```python
from build123d import *

# Parameters (mm, degrees)
SKETCH_1_W      = 14.7
SKETCH_1_H      = 5.8
EXTRUDE_1_DEPTH = 6


with BuildPart() as part:
    # Эскиз1 → Бобышка-Вытянуть1 (new body)
    with BuildSketch(Plane.XY):
        Polygon((-327.15, -30.4), (327.15, -30.4), (327.15, -17.066666667), (330.45862, -17.066666667), (330.45862, -6.666666667), (327.15, -6.666666667), (327.15, 6.666666667), (330.45862, 6.666666667), (330.45862, 17.066666667), (327.15, 17.066666667), (327.15, 30.4), (-327.15, 30.4), (-330.45862, 30.4), (-330.45862, 16.533333333), (-327.15, 16.533333333), (-327.15, 6.933333333), (-330.45862, 6.933333333), (-330.45862, -6.933333333), (-327.15, -6.933333333), (-327.15, -16.533333333), (-330.45862, -16.533333333), (-330.45862, -30.4), align=None)
        with Locations((-252.05, -2.5)):
            Rectangle(SKETCH_1_W, SKETCH_1_H, mode=Mode.SUBTRACT)
        with Locations((-302.46, -2.5)):
            Rectangle(SKETCH_1_W, SKETCH_1_H, mode=Mode.SUBTRACT)
        with Locations((-201.64, -2.5)):
            Rectangle(SKETCH_1_W, SKETCH_1_H, mode=Mode.SUBTRACT)
        with Locations((-151.23, -2.5)):
            Rectangle(SKETCH_1_W, SKETCH_1_H, mode=Mode.SUBTRACT)
        with Locations((-100.82, -2.5)):
            Rectangle(SKETCH_1_W, SKETCH_1_H, mode=Mode.SUBTRACT)
        with Locations((-50.41, -2.5)):
            Rectangle(SKETCH_1_W, SKETCH_1_H, mode=Mode.SUBTRACT)
        with Locations((0, -2.5)):
            Rectangle(SKETCH_1_W, SKETCH_1_H, mode=Mode.SUBTRACT)
        with Locations((50.41, -2.5)):
            Rectangle(SKETCH_1_W, SKETCH_1_H, mode=Mode.SUBTRACT)
        with Locations((100.82, -2.5)):
            Rectangle(SKETCH_1_W, SKETCH_1_H, mode=Mode.SUBTRACT)
        with Locations((151.23, -2.5)):
            Rectangle(SKETCH_1_W, SKETCH_1_H, mode=Mode.SUBTRACT)
        with Locations((201.64, -2.5)):
            Rectangle(SKETCH_1_W, SKETCH_1_H, mode=Mode.SUBTRACT)
        with Locations((252.05, -2.5)):
            Rectangle(SKETCH_1_W, SKETCH_1_H, mode=Mode.SUBTRACT)
        with Locations((302.46, -2.5)):
            Rectangle(SKETCH_1_W, SKETCH_1_H, mode=Mode.SUBTRACT)
    extrude(amount=EXTRUDE_1_DEPTH)


solid = part.part
```
Part model, mm, in its own coordinate system. Round coordinates to 2 decimals unless told otherwise and drop trailing zeros. One line per question, with ' | ' between items.
(1) Probe line 1 along Y through (x, z) = (-152, 3.4); line 2 along X through (y, z) = (-14, 4); line 3 along X through (y, z) = (-22, 4.55). List the from-to ranges inside material, lowest first.
Answer key:
line 1: y = -30.4 to -5.4, 0.4 to 30.4 | line 2: x = -327.15 to 330.46 | line 3: x = -330.46 to 327.15
(2) Saw through at A-A on z = 2.6. Count the separate pieces of the cut face and the enclosed holes in it, then the cut area to 3 significant figures.
Answer key:
separate pieces: 1 | enclosed holes: 13 | area: 38,900 mm^2
(3) Pin check, flat tips, straight feed: pin 1 (2.5 mm diameter, centred on x = 328.5, z = 4, fed in from -Y); pin 2 (3 mm diameter, centred on y = -2.5, z = 3, fed in from +X); pin 3 (3 mm diameter, centred on y = 9.5, z = 3, fed in from -X). Stop position of each tip, or through.
Answer key:
pin 1: stops at y = -17.07 | pin 2: stops at x = 327.15 | pin 3: stops at x = -327.15
